For this review, take the finished solid that the model builds, in its own axes (mm). Face numbers are marked on the shaded views. A direction names the side the tool comes from. Round coordinates to 2 decimals unless told otherwise and drop trailing zeros. Write each loop counter-clockwise with the first axis right and the second up, starting at its lowest first coordinate (ties: lowest second). Pieces come first, ordered by that corner, then holes. Notation, with made-up numbers: (14.25, 68.5) -> (47.25, 68.5) arc R13 ccw to (47.25, 91.5) -> close; hole circle Ø4 at (57.25, 63.5). An arc over 180 degrees is marked (long way). Answer as CSV lines item,"result". Start each with the question number.
Item 1: For pin 1 Ø7 at (x, z) = (-21.03, 57.37) entering from -Y; pin 2 Ø5 at (x, y) = (-40.5, -24) entering from -Z (3 decimals); pin 3 Ø4 at (x, z) = (14.33, 57.37) entering from +Y; pin 4 Ø11 at (x, z) = (-36, 23.5) entering from +Y, all flat-tipped, find the tip position at first contact; note any pin that passes through.
Item 2: Take a section at B-B on x = 0. Give the boundary of the cut face in (y, z), then the cut area to 3 significant figures.
Item 3: Wall thickness on probe 1 along Y at (x, z) = (0, 2); probe 2 along X at (y, z) = (-41.5, 51); probe 3 along Y at (x, z) = (-39, 8.5): over which ranges is each line inside the solid? List them lowest first. Write a range as from..to.
Item 4: Take a section at C-C on z = 42. Give the boundary of the cut face in (x, y), then the cut area to 3 significant figures.
Item 5: Machinability: for the marked faces 1, 2 and 3, which of the approach directions +Z, -Z, +X, -X, +Y, -Y give a long, thin tool a straight path to every point of the face, cutting with its end or side? Answer none if there is none.
Item 6: Take a section at D-D on z = 31.5. Give the boundary of the cut face in (x, y), then the cut area to 3 significant figures.
```python
from build123d import *

# Parameters (mm, degrees)
SKETCH1_R           = 33.3375
SKETCH1_R_2         = 2.25
SKETCH1_R_3         = 1.65
SKETCH1_R_4         = 20.6375
BOSS_EXTRUDE1_DEPTH = 6.35
BOSS_EXTRUDE3_DEPTH = 6.35
SKETCH4_R           = 33.3375
SKETCH4_R_2         = 2.25
SKETCH4_R_3         = 1.65
SKETCH4_R_4         = 20.6375
BOSS_EXTRUDE4_DEPTH = 6.35
FILLET1_R           = 12.7
FILLET2_R           = 12.7
FILLET3_R           = 12.7


with BuildPart() as part:
    # Sketch1 → Boss-Extrude1 (new body)
    # profile 1 of 2: a face of its own
    with BuildSketch(Plane.XY):
        Circle(SKETCH1_R)
        with Locations((-17.67766953, 17.67766953)):
            Circle(SKETCH1_R_2, mode=Mode.SUBTRACT)
        with Locations((17.67766953, 17.67766953)):
            Circle(SKETCH1_R_3, mode=Mode.SUBTRACT)
        with Locations((17.67766953, -17.67766953)):
            Circle(SKETCH1_R_2, mode=Mode.SUBTRACT)
        with Locations((-17.67766953, -17.67766953)):
            Circle(SKETCH1_R_3, mode=Mode.SUBTRACT)
        Circle(SKETCH1_R_4, mode=Mode.SUBTRACT)
    # profile 2 of 2: a face of its own
    with BuildSketch(Plane.XY):
        with BuildLine():
            ThreePointArc((-30.823674444, -12.7), (-33.3375, 0), (-30.823674444, 12.7))
            Line((-30.823674444, 12.7), (-38.1, 12.7))
            Line((-38.1, 12.7), (-38.1, -12.7))
            Line((-38.1, -12.7), (-30.823674444, -12.7))
        make_face()
    extrude(amount=BOSS_EXTRUDE1_DEPTH)

    # Sketch2 → Boss-Extrude3 (add)
    with BuildSketch(Plane.ZY.offset(38.1)):
        Polygon((0, 12.7), (57.15, 12.7), (57.15, -88.9), (22.225, -88.9), (22.225, -12.7), (0, -12.7), align=None)
        with BuildLine():
            Line((46.0375, -6.35), (46.0375, -69.85))
            ThreePointArc((46.0375, -69.85), (39.6875, -76.2), (33.3375, -69.85))
            Line((33.3375, -69.85), (33.3375, -6.35))
            ThreePointArc((33.3375, -6.35), (39.6875, 0), (46.0375, -6.35))
        make_face(mode=Mode.SUBTRACT)
    extrude(amount=BOSS_EXTRUDE3_DEPTH)

    # Sketch4 → Boss-Extrude4 (add)
    # profile 1 of 2: a face of its own
    with BuildSketch(Plane(origin=(0, -88.9, 0), x_dir=(-1, 0, 0), z_dir=(0, -1, 0))):
        with BuildLine():
            ThreePointArc((36.689436686, -39.6875), (35.430818695, -48.761321425), (31.75, -57.15))
            Line((31.75, -57.15), (44.45, -57.15))
            Line((44.45, -57.15), (44.45, -22.225))
            Line((44.45, -22.225), (31.75, -22.225))
            ThreePointArc((31.75, -22.225), (35.430818695, -30.613678575), (36.689436686, -39.6875))
        make_face()
    # profile 2 of 2: a face of its own
    with BuildSketch(Plane(origin=(0, -88.9, 0), x_dir=(-1, 0, 0), z_dir=(0, -1, 0))):
        with Locations((3.351936686, -39.6875)):
            Circle(SKETCH4_R)
        with Locations(Location((21.029606215, -57.36516953, 0), (0, 0, 90))):
            Circle(SKETCH4_R_2, mode=Mode.SUBTRACT)
        with Locations(Location((-14.325732844, -57.36516953, 0), (0, 0, 90))):
            Circle(SKETCH4_R_3, mode=Mode.SUBTRACT)
        with Locations(Location((-14.325732844, -22.00983047, 0), (0, 0, 90))):
            Circle(SKETCH4_R_2, mode=Mode.SUBTRACT)
        with Locations(Location((21.029606215, -22.00983047, 0), (0, 0, 90))):
            Circle(SKETCH4_R_3, mode=Mode.SUBTRACT)
        with Locations(Location((3.351936686, -39.6875, 0), (0, 0, 90))):
            Circle(SKETCH4_R_4, mode=Mode.SUBTRACT)
    extrude(amount=BOSS_EXTRUDE4_DEPTH)

    # Fillet1
    fillet1_edges = [part.edges().sort_by_distance(p)[0] for p in [
        (-44.45, 0, 0),
    ]]
    fillet(fillet1_edges, radius=FILLET1_R)

    # Fillet2
    fillet2_edges = [part.edges().sort_by_distance(p)[0] for p in [
        (-44.45, -95.25, 39.6875),
    ]]
    fillet(fillet2_edges, radius=FILLET2_R)

    # Fillet3
    fillet3_edges = [part.edges().sort_by_distance(p)[0] for p in [
        (-41.275, 12.7, 57.15),
    ]]
    fillet(fillet3_edges, radius=FILLET3_R)


solid = part.part
```
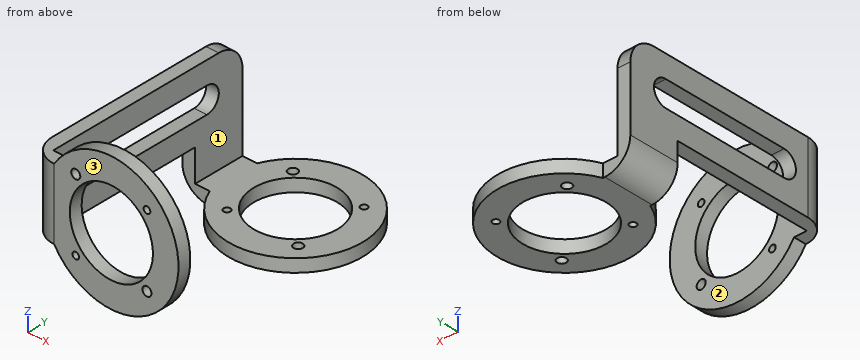
Output values:
1,pin 1,"stops at y = -95.25"
1,pin 2,"stops at z = 22.225"
1,pin 3,"stops at y = -88.9"
1,pin 4,"stops at y = 12.7"
2,outline,"(-95.25, 6.52) -> (-88.9, 6.52) -> (-88.9, 19.32) -> (-95.25, 19.32) -> close; (-95.25, 60.05) -> (-88.9, 60.05) -> (-88.9, 72.86) -> (-95.25, 72.86) -> close; (-33.34, 0) -> (-20.64, 0) -> (-20.64, 6.35) -> (-33.34, 6.35) -> close; (20.64, 0) -> (33.34, 0) -> (33.34, 6.35) -> (20.64, 6.35) -> close"
2,area,"324 mm^2"
3,probe 1,"y = -33.34..-20.64, 20.64..33.34"
3,probe 2,"x = -44.45..-38.1"
3,probe 3,"y = -12.7..12.7"
4,outline,"(-44.45, -82.55) arc R12.7 ccw to (-31.75, -95.25) -> (-23.86, -95.25) -> (-23.86, -88.9) -> (-38.1, -88.9) -> (-38.1, -75.76) -> (-44.45, -75.76) -> close; (-44.45, -0.44) -> (-38.1, -0.44) -> (-38.1, 12.7) -> (-44.45, 12.7) -> close; (17.16, -95.25) -> (29.91, -95.25) -> (29.91, -88.9) -> (17.16, -88.9) -> close"
4,area,"344 mm^2"
5,face 1,"+Z, +X, +Y"
5,face 2,"+Z, -Z, +X, +Y"
5,face 3,"+Z, -Z, +X, -X, -Y"
6,outline,"(-44.45, -82.55) arc R12.7 ccw to (-31.75, -95.25) -> (-22.3, -95.25) -> (-22.3, -88.9) -> (-38.1, -88.9) -> (-38.1, 12.7) -> (-44.45, 12.7) -> close; (15.59, -95.25) -> (28.96, -95.25) -> (28.96, -88.9) -> (15.59, -88.9) -> close"
6,area,"836 mm^2"
